from build123d import *

# Parameters (mm, degrees)
SKETCH1_W           = 88
SKETCH1_H           = 88
BOSS_EXTRUDE1_DEPTH = 2
FILLET1_R           = 2
SKETCH2_R           = 1.85
CUT_EXTRUDE1_DEPTH  = 10
SKETCH3_R           = 1.85
CUT_EXTRUDE2_DEPTH  = 5


with BuildPart() as part:
    # Sketch1 → Boss-Extrude1 (new body)
    with BuildSketch(Plane(origin=(0, 0, 0), x_dir=(1, 0, 0), z_dir=(0, 1, 0))):
        Rectangle(SKETCH1_W, SKETCH1_H)
    extrude(amount=BOSS_EXTRUDE1_DEPTH)

    # Fillet1
    fillet1_edges = [part.edges().sort_by_distance(p)[0] for p in [
        (-44, 1, -44),
        (44, 1, -44),
        (44, 1, 44),
        (-44, 1, 44),
    ]]
    fillet(fillet1_edges, radius=FILLET1_R)

    # Sketch2 → Cut-Extrude1 (cut)
    with BuildSketch(Plane.XZ):
        with Locations(Location((-32, 38.82, 0), (0, 0, 270))):
            Circle(SKETCH2_R)
        with Locations(Location((32, 38.82, 0), (0, 0, 270))):
            Circle(SKETCH2_R)
        with Locations(Location((32, -38.82, 0), (0, 0, 270))):
            Circle(SKETCH2_R)
        with Locations(Location((-32, -38.82, 0), (0, 0, 270))):
            Circle(SKETCH2_R)
    extrude(amount=-CUT_EXTRUDE1_DEPTH, mode=Mode.SUBTRACT)

    # Sketch3 → Cut-Extrude2 (cut)
    with BuildSketch(Plane.XZ):
        with Locations(Location((-34.25, 10.7, 0), (0, 0, 270))):
            Circle(SKETCH3_R)
        with Locations(Location((0, 10.7, 0), (0, 0, 270))):
            Circle(SKETCH3_R)
        with Locations(Location((34.25, 10.7, 0), (0, 0, 270))):
            Circle(SKETCH3_R)
        with Locations(Location((34.25, -16.7, 0), (0, 0, 270))):
            Circle(SKETCH3_R)
        with Locations(Location((0, -16.7, 0), (0, 0, 270))):
            Circle(SKETCH3_R)
        with Locations(Location((-34.25, -16.7, 0), (0, 0, 270))):
            Circle(SKETCH3_R)
    extrude(amount=-CUT_EXTRUDE2_DEPTH, mode=Mode.SUBTRACT)


solid = part.part
For this review, take the finished solid that the model builds, in its own axes (mm). Give positions to 0.01 mm unless a question says otherwise; leave off trailing zeros. Loops run counter-clockwise (first coordinate to the right, second up) from the corner with the lowest first, then second, coordinate; pieces in that order, holes last. Notation, with made-up numbers: (89, 11.25) - (133, 11.25) arc R17 ccw to (133, 44.25) - close; hole circle Ø3 at (-6.75, 45.25). An arc over 180 degrees is marked (long way). Write each question's results on one line, items separated by ' | '.
(1) Take a section at B-B (z = -38.82). Give the boundary of the cut face in (x, y).
Conclusion:
outline: (-44, 0) - (-33.85, 0) - (-33.85, 2) - (-44, 2) - close; (-30.15, 0) - (30.15, 0) - (30.15, 2) - (-30.15, 2) - close; (33.85, 0) - (44, 0) - (44, 2) - (33.85, 2) - close
(2) For line 1 along X through (y, z) = (1.05, 10.7); line 2 along X through (y, z) = (0.6, 38.82); line 3 along X through (y, z) = (0.3, -40), list the stretches that pass through material, from the lowest coordinate up.
Conclusion:
line 1: -44 to -36.1, -32.4 to -1.85, 1.85 to 32.4, 36.1 to 44 | line 2: -44 to -33.85, -30.15 to 30.15, 33.85 to 44 | line 3: -44 to -33.42, -30.58 to 30.58, 33.42 to 44
(3) Take a section at A-A (x = 0). Give the boundary of the cut face in (y, z).
Conclusion:
outline: (0, -44) - (2, -44) - (2, -18.55) - (0, -18.55) - close; (0, -14.85) - (2, -14.85) - (2, 8.85) - (0, 8.85) - close; (0, 12.55) - (2, 12.55) - (2, 44) - (0, 44) - close
(4) Draft analysis for pull direction X (two halves, no side actions). For faces 1 (the cylindrical face through (-43.43, 1.01, -43.4)), 2 (the cylindrical face through (-32.69, 0.986, 9.705)), 3 (the flat face through (-1, 2, -1)), state which applies: +X half, -X half, draft (parallel to the pull), parting line (faces both ways), or undercut.
Conclusion:
face 1: -X half | face 2: undercut | face 3: draft
(5) For pin 1 Ø3.5 at (x, z) = (32, -38.82) entering from +Y, flat-tipped, find the tip position at first contact; note if it passes through.
Conclusion:
pin 1: through
(6) Take a section at C-C (z = 10.7). Give the boundary of the cut face in (x, y).
Conclusion:
outline: (-44, 0) - (-36.1, 0) - (-36.1, 2) - (-44, 2) - close; (-32.4, 0) - (-1.85, 0) - (-1.85, 2) - (-32.4, 2) - close; (1.85, 0) - (32.4, 0) - (32.4, 2) - (1.85, 2) - close; (36.1, 0) - (44, 0) - (44, 2) - (36.1, 2) - close
